Source: CAD feature listing. Evaluate the final solid. Frame: model axes, mm. A direction names the side the tool comes from. Give positions to 0.01 mm unless a question says otherwise; leave off trailing zeros. Order: outer loops, then holes, each group sorted by start corner. A loop starts at its lowest first (then second) coordinate and runs counter-clockwise, first axis right, second up. Notation, with made-up numbers: (-9, 84) -> (27, 84) arc R31 cw to (27, 113) -> close; hole circle Ø9 at (-16, 68.5). An arc over 180 degrees is marked (long way). Use one line per item in the form item = value. Start each with the question number.
from build123d import *

# Parameters (mm, degrees)
SKETCH1_W           = 180
SKETCH1_H           = 70
BOSS_EXTRUDE1_DEPTH = 10
SKETCH2_R           = 1.5
CUT_EXTRUDE1_DEPTH  = 5
FILLET1_R           = 2
SHELL1_START        = 2
SHELL1_OUTLINE_W    = 176
SHELL1_OUTLINE_H    = 66
SHELL1_OUTLINE_R    = 3.5
SHELL1_DEPTH        = 8
SHELL1_START_2      = 7
SHELL1_2_OUTLINE_R  = 3.5
SHELL1_2_DEPTH      = 3


# Read off the part's stored shape, not the designer's step: Shell1
with BuildPart() as part:
    # Sketch1 → Boss-Extrude1 (new body)
    with BuildSketch(Plane(origin=(0, 0, 0), x_dir=(1, 0, 0), z_dir=(0, 1, 0))):
        Rectangle(SKETCH1_W, SKETCH1_H)
    extrude(amount=BOSS_EXTRUDE1_DEPTH)

    # Sketch2 → Cut-Extrude1 (cut)
    with BuildSketch(Plane.XZ):
        with Locations(Location((50, 0, 0), (0, 0, 270))):
            Circle(SKETCH2_R)
    cut_extrude1 = extrude(amount=-CUT_EXTRUDE1_DEPTH, mode=Mode.SUBTRACT)

    # Mirror1: Cut-Extrude1 across plane
    add(cut_extrude1.mirror(Plane(origin=(0, 0, 0), x_dir=(0, 0, 1), z_dir=(1, 0, 0))), mode=Mode.SUBTRACT)

    # Fillet1
    fillet1_edges = [part.edges().sort_by_distance(p)[0] for p in [
        (-90, 10, 0),
        (0, 10, 35),
        (90, 10, 0),
        (0, 0, 35),
        (-90, 0, 0),
        (0, 0, -35),
        (90, 0, 0),
        (90, 5, 35),
        (-90, 5, 35),
        (-90, 5, -35),
        (90, 5, -35),
        (0, 10, -35),
    ]]
    fillet(fillet1_edges, radius=FILLET1_R)

    # Shell1 outline → Shell1 (cut)
    with BuildSketch(Plane(origin=(0, 0, 0), x_dir=(1, 0, 0), z_dir=(0, 1, 0)).offset(SHELL1_START)):
        Rectangle(SHELL1_OUTLINE_W, SHELL1_OUTLINE_H)
        with Locations((-50, 0)):
            Circle(SHELL1_OUTLINE_R, mode=Mode.SUBTRACT)
        with Locations((50, 0)):
            Circle(SHELL1_OUTLINE_R, mode=Mode.SUBTRACT)
    extrude(amount=SHELL1_DEPTH, mode=Mode.SUBTRACT)

    # Shell1 2 outline → Shell1 2 (cut)
    with BuildSketch(Plane(origin=(0, 0, 0), x_dir=(1, 0, 0), z_dir=(0, 1, 0)).offset(SHELL1_START_2)):
        with Locations((50, 0)):
            Circle(SHELL1_2_OUTLINE_R)
        with Locations((-50, 0)):
            Circle(SHELL1_2_OUTLINE_R)
    extrude(amount=SHELL1_2_DEPTH, mode=Mode.SUBTRACT)


solid = part.part
1) Pin query (flat end, axial travel): pin 1 (1.5 mm diameter, centred on x = -50.5, z = 0, fed in from -Y); pin 2 (3.5 mm diameter, centred on x = -48.5, z = 0.5, fed in from +Y); pin 3 (10 mm diameter, centred on x = -31, z = 5.5, fed in from +Y). Return the tip coordinate at first contact, or that it passes through.
2) Draft query along X for faces 1 (the face through (50, 7, 0)), 2 (the face through (-1, 5, -35)), 3 (the face through (-90, 5, 0)), 4 (the face through (50, 5, 0)). Return one class per face: +X half, -X half, draft (parallel to the pull), parting line (faces both ways), or undercut.
3) Cut plane A-A, the plane z = 19. Return the cut outline in (x, y).
4) Material intervals for probe 1 along X at (y, z) = (3.4, 0); probe 2 along Z at (x, y) = (-50, 4.05); probe 3 along X at (y, z) = (5.75, 23), sorted ascending.
5) Cut plane B-B, the plane x = 73. Return the cut outline in (y, z), plus the area to 3 significant figures.
6) Reachability of faces 5 (the face through (-1, 0, 0)), 6 (the face through (-53.497, 4.465, -0.154)), 7 (the face through (-48.536, 2.465, 0.325)) from +Z, -Z, +X, -X, +Y, -Y: full face, straight path, thin tool, end or side. Return the list, or none.
Output values:
q1.pin_1 = 5
q1.pin_2 = 7
q1.pin_3 = 2
q2.face_1 = undercut
q2.face_2 = draft
q2.face_3 = -X half
q2.face_4 = undercut
q3.outline = (-90, 2) arc R2 ccw to (-88, 0) -> (88, 0) arc R2 ccw to (90, 2) -> (90, 8) arc R2 ccw to (88, 10) -> (88, 2) -> (-88, 2) -> (-88, 10) arc R2 ccw to (-90, 8) -> close
q4.probe_1 = -90 to -88, -53.5 to -51.5, -48.5 to -46.5, 46.5 to 48.5, 51.5 to 53.5, 88 to 90
q4.probe_2 = -35 to -33, -3.5 to -1.5, 1.5 to 3.5, 33 to 35
q4.probe_3 = -90 to -88, 88 to 90
q5.outline = (0, -33) arc R2 ccw to (2, -35) -> (8, -35) arc R2 ccw to (10, -33) -> (2, -33) -> (2, 33) -> (10, 33) arc R2 ccw to (8, 35) -> (2, 35) arc R2 ccw to (0, 33) -> close
q5.area = 169 mm^2
q6.face_5 = +Z, -Z, +X, -X, -Y
q6.face_6 = +Y
q6.face_7 = -Y
